Geometry: final body of the model. Coordinates: model frame, mm. A direction names the side the tool comes from. Round coordinates to 2 decimals unless told otherwise and drop trailing zeros. Write each loop counter-clockwise with the first axis right and the second up, starting at its lowest first coordinate (ties: lowest second). Pieces come first, ordered by that corner, then holes. Notation, with made-up numbers: (-38.75, 80) -> (-9.75, 80) arc R25 cw to (-9.75, 96) -> close; hole circle Ø11 at (-11.5, 77). An arc over 180 degrees is marked (long way). Use one line per item in the form item = value. Start each with the question number.
1. Draft query along Y for faces 1 (the face through (-23.476, 6.141, 0.14)), 2 (the face through (-45, 4, 0)), 3 (the face through (-30, 7.25, 0)). Return one class per face: pulls with the +Y half, pulls with the -Y half, needs draft (parallel to the pull), parting line crosses it, or undercut.
2. Pin query (flat end, axial travel): pin 1 Ø4 at (y, z) = (20, 3.5) entering from +X; pin 2 Ø7.5 at (x, z) = (-2, -4.5) entering from -Y; pin 3 Ø1.5 at (x, z) = (-23.5, -2) entering from -Y; pin 4 Ø17 at (x, y) = (30, 50) entering from +Z. Return the tip coordinate at first contact, or that it passes through.
3. Cut plane A-A, the plane x = 30. Return the cut outline in (y, z).
4. Cut plane B-B, the plane y = 15. Return the cut outline in (x, z), plus the area to 3 significant figures.
5. Reachability of faces 4 (the face through (-43.8, 21.3, 0.1)), 5 (the face through (6.524, 6.141, 0.14)), 6 (the face through (30, 7.25, 0)) from +Z, -Z, +X, -X, +Y, -Y: full face, straight path, thin tool, end or side. Return the list, or none.
6. Cut plane D-D, the plane y = 50. Return the cut outline in (x, z).
7. Line query: L1, parallel to Y at x = 12, z = 4; L2, parallel to X at y = 17.5, z = 5.5; L3, parallel to X at y = 39, z = -8.5. Output: solid intervals per line, ascending.
8. Cut plane C-C, the plane y = 62. Return the cut outline in (x, z), plus the area to 3 significant figures.
```python
from build123d import *

# Parameters (mm, degrees)
SKETCH1_R           = 5.25
SKETCH1_R_2         = 8
SKETCH1_R_3         = 9.5
SKETCH1_R_4         = 3.75
BOSS_EXTRUDE1_DEPTH = 10


with BuildPart() as part:
    # Sketch1 → Boss-Extrude1 (new, symmetric)
    with BuildSketch(Plane.XY):
        Polygon((45, 70), (-45, 70), (-45, 22.5), (-42.5, 20), (-42.5, 23.5), (-40, 23.5), (-37.75, 19.602885683), (-37.75, 10.397114317), (-40, 6.5), (-42.5, 6.5), (-42.5, 10), (-45, 7.5), (-45, 0), (-37.5, 0), (-35, 2.5), (-38.5, 2.5), (-38.5, 5), (-34.602885683, 7.25), (-25.397114317, 7.25), (-21.5, 5), (-21.5, 2.5), (-25, 2.5), (-22.5, 0), (-7.5, 0), (-5, 2.5), (-8.5, 2.5), (-8.5, 5), (-4.602885683, 7.25), (4.602885683, 7.25), (8.5, 5), (8.5, 2.5), (5, 2.5), (7.5, 0), (22.5, 0), (25, 2.5), (21.5, 2.5), (21.5, 5), (25.397114317, 7.25), (34.602885683, 7.25), (38.5, 5), (38.5, 2.5), (35, 2.5), (37.5, 0), (45, 0), (45, 7.5), (42.5, 10), (42.5, 6.5), (40, 6.5), (37.75, 10.397114317), (37.75, 19.602885683), (40, 23.5), (42.5, 23.5), (42.5, 20), (45, 22.5), align=None)
        with Locations((0, 15)):
            Circle(SKETCH1_R, mode=Mode.SUBTRACT)
        with Locations((-30, 15)):
            Circle(SKETCH1_R, mode=Mode.SUBTRACT)
        with Locations((30, 15)):
            Circle(SKETCH1_R, mode=Mode.SUBTRACT)
        with Locations((0, 50)):
            Circle(SKETCH1_R_2, mode=Mode.SUBTRACT)
        with Locations((30, 50)):
            Circle(SKETCH1_R_3, mode=Mode.SUBTRACT)
        with Locations((12, 62)):
            Circle(SKETCH1_R_4, mode=Mode.SUBTRACT)
        with Locations((12, 38)):
            Circle(SKETCH1_R_4, mode=Mode.SUBTRACT)
        with Locations((-12, 38)):
            Circle(SKETCH1_R_4, mode=Mode.SUBTRACT)
        with Locations((-12, 62)):
            Circle(SKETCH1_R_4, mode=Mode.SUBTRACT)
        with Locations((-30, 50)):
            Circle(SKETCH1_R_3, mode=Mode.SUBTRACT)
    extrude(amount=BOSS_EXTRUDE1_DEPTH, both=True)


solid = part.part
```
Outcome:
q1.face_1 = undercut
q1.face_2 = needs draft
q1.face_3 = pulls with the -Y half
q2.pin_1 = 44.5
q2.pin_2 = 1.75
q2.pin_3 = 0.25
q2.pin_4 = through
q3.outline = (7.25, -10) -> (9.75, -10) -> (9.75, 10) -> (7.25, 10) -> close; (20.25, -10) -> (40.5, -10) -> (40.5, 10) -> (20.25, 10) -> close; (59.5, -10) -> (70, -10) -> (70, 10) -> (59.5, 10) -> close
q4.outline = (-37.75, -10) -> (-35.25, -10) -> (-35.25, 10) -> (-37.75, 10) -> close; (-24.75, -10) -> (-5.25, -10) -> (-5.25, 10) -> (-24.75, 10) -> close; (5.25, -10) -> (24.75, -10) -> (24.75, 10) -> (5.25, 10) -> close; (35.25, -10) -> (37.75, -10) -> (37.75, 10) -> (35.25, 10) -> close
q4.area = 880 mm^2
q5.face_4 = +Z, -Z, -X
q5.face_5 = +Z, -Z
q5.face_6 = +Z, -Z, -Y
q6.outline = (-45, -10) -> (-39.5, -10) -> (-39.5, 10) -> (-45, 10) -> close; (-20.5, -10) -> (-8, -10) -> (-8, 10) -> (-20.5, 10) -> close; (8, -10) -> (20.5, -10) -> (20.5, 10) -> (8, 10) -> close; (39.5, -10) -> (45, -10) -> (45, 10) -> (39.5, 10) -> close
q7.L1 = 0 to 34.25, 41.75 to 58.25, 65.75 to 70
q7.L2 = -37.75 to -34.62, -25.38 to -4.62, 4.62 to 25.38, 34.62 to 37.75
q7.L3 = -45 to -15.61, -8.39 to 8.39, 15.61 to 45
q8.outline = (-45, -10) -> (-15.75, -10) -> (-15.75, 10) -> (-45, 10) -> close; (-8.25, -10) -> (8.25, -10) -> (8.25, 10) -> (-8.25, 10) -> close; (15.75, -10) -> (45, -10) -> (45, 10) -> (15.75, 10) -> close
q8.area = 1,500 mm^2
